```python
from build123d import *

# Parameters (mm, degrees)
SKETCH1_W                          = 165.1
SKETCH1_H                          = 12.7
BOSS_EXTRUDE1_DEPTH                = 127
SKETCH2_R                          = 30.63494
CUT_EXTRUDE1_DEPTH                 = 153.002606886
SKETCH3_R                          = 31.75
CUT_EXTRUDE2_DEPTH                 = 7.62
CUT_EXTRUDE3_DEPTH                 = 153.002606886
FILLET1_R                          = 3.175
FILLET2_R                          = 1.5875
SKETCH5_W                          = 101.6
SKETCH5_H                          = 9.525
CUT_EXTRUDE4_DEPTH                 = 153.002606886
FILLET3_R                          = 3.175
F_1_16_0_0625_DIAMETER_HOLE1_D     = 1.5875
F_1_16_0_0625_DIAMETER_HOLE1_DEPTH = 15.875
F_1_16_0_0625_DIAMETER_HOLE1_TIP   = 0.476933116
F_1_16_0_0625_DIAMETER_HOLE2_D     = 1.5875
F_1_16_0_0625_DIAMETER_HOLE2_DEPTH = 15.875
F_1_16_0_0625_DIAMETER_HOLE2_TIP   = 0.476933116
CUT_EXTRUDE5_DEPTH                 = 153.002606886


with BuildPart() as part:
    # Sketch1 → Boss-Extrude1 (new, symmetric)
    with BuildSketch(Plane(origin=(0, 0, 0), x_dir=(1, 0, 0), z_dir=(0, 1, 0))):
        Rectangle(SKETCH1_W, SKETCH1_H)
    extrude(amount=BOSS_EXTRUDE1_DEPTH, both=True)

    # Sketch2 → Cut-Extrude1 (cut, through all)
    with BuildSketch(Plane.XY.offset(6.35)):
        with Locations((0, 127)):
            Circle(SKETCH2_R)
    extrude(amount=-CUT_EXTRUDE1_DEPTH, mode=Mode.SUBTRACT)

    # Sketch3 → Cut-Extrude2 (cut)
    with BuildSketch(Plane(origin=(0, 0, -6.35), x_dir=(-1, 0, 0), z_dir=(0, 0, -1))):
        with Locations((0, 127)):
            Circle(SKETCH3_R)
    extrude(amount=-CUT_EXTRUDE2_DEPTH, mode=Mode.SUBTRACT)

    # Sketch4 → Cut-Extrude3 (cut, through all)
    with BuildSketch(Plane.XY.offset(6.35)):
        with BuildLine():
            Line((57.277, 127), (57.277, 104.775))
            Line((57.277, 104.775), (43.877983689, 104.775))
            Line((43.877983689, 104.775), (38.415383769, 114.236500603))
            ThreePointArc((38.415383769, 114.236500603), (39.624000301, 118.747116057), (44.134615883, 117.5385))
            Line((44.134615883, 117.5385), (47.690804866, 111.379))
            Line((47.690804866, 111.379), (50.673, 111.379))
            Line((50.673, 111.379), (50.673, 127))
            Line((50.673, 127), (57.277, 127))
        make_face()
        with BuildLine():
            Line((-50.673, 127), (-57.277, 127))
            Line((-57.277, 127), (-57.277, 104.775))
            Line((-57.277, 104.775), (-43.877983689, 104.775))
            Line((-43.877983689, 104.775), (-38.415383769, 114.236500603))
            ThreePointArc((-38.415383769, 114.236500603), (-39.624000301, 118.747116057), (-44.134615883, 117.5385))
            Line((-44.134615883, 117.5385), (-47.690804866, 111.379))
            Line((-47.690804866, 111.379), (-50.673, 111.379))
            Line((-50.673, 111.379), (-50.673, 127))
        make_face()
    extrude(amount=-CUT_EXTRUDE3_DEPTH, mode=Mode.SUBTRACT)

    # Fillet1
    fillet1_edges = [part.edges().sort_by_distance(p)[0] for p in [
        (50.673, 127, 0),
        (57.277, 127, 0),
        (57.277, 104.775, 0),
        (43.877983689, 104.775, 0),
        (-43.877983689, 104.775, 0),
        (-57.277, 104.775, 0),
        (-57.277, 127, 0),
        (-50.673, 127, 0),
    ]]
    fillet(fillet1_edges, radius=FILLET1_R)

    # Fillet2
    fillet2_edges = [part.edges().sort_by_distance(p)[0] for p in [
        (47.690804866, 111.379, 0),
        (50.673, 111.379, 0),
        (-50.673, 111.379, 0),
        (-47.690804866, 111.379, 0),
    ]]
    fillet(fillet2_edges, radius=FILLET2_R)

    # Sketch5 → Cut-Extrude4 (cut, through all)
    with BuildSketch(Plane.XY.offset(6.35)):
        with Locations((0, -122.2375)):
            Rectangle(SKETCH5_W, SKETCH5_H)
    extrude(amount=-CUT_EXTRUDE4_DEPTH, mode=Mode.SUBTRACT)

    # Fillet3
    fillet3_edges = [part.edges().sort_by_distance(p)[0] for p in [
        (-50.8, -127, 0),
        (-50.8, -117.475, 0),
        (50.8, -117.475, 0),
        (50.8, -127, 0),
    ]]
    fillet(fillet3_edges, radius=FILLET3_R)

    # 1/16 (0.0625) Diameter Hole1
    with Locations(Plane(origin=(82.55, 0, 0), x_dir=(0, 0, -1), z_dir=(1, 0, 0))):
        with Locations((0, -120.65), (0, -95.25), (0, 44.45), (0, 69.85), (0, 120.65)):
            Hole(F_1_16_0_0625_DIAMETER_HOLE1_D / 2, depth=F_1_16_0_0625_DIAMETER_HOLE1_DEPTH)
            with Locations((0, 0, -(F_1_16_0_0625_DIAMETER_HOLE1_DEPTH + F_1_16_0_0625_DIAMETER_HOLE1_TIP / 2))):  # 118° drill point
                Cone(0, F_1_16_0_0625_DIAMETER_HOLE1_D / 2, F_1_16_0_0625_DIAMETER_HOLE1_TIP, mode=Mode.SUBTRACT)

    # 1/16 (0.0625) Diameter Hole2
    with Locations(Plane.ZY.offset(82.55)):
        with Locations((0, -120.65), (0, -95.25), (0, 44.45), (0, 69.85), (0, 120.65)):
            Hole(F_1_16_0_0625_DIAMETER_HOLE2_D / 2, depth=F_1_16_0_0625_DIAMETER_HOLE2_DEPTH)
            with Locations((0, 0, -(F_1_16_0_0625_DIAMETER_HOLE2_DEPTH + F_1_16_0_0625_DIAMETER_HOLE2_TIP / 2))):  # 118° drill point
                Cone(0, F_1_16_0_0625_DIAMETER_HOLE2_D / 2, F_1_16_0_0625_DIAMETER_HOLE2_TIP, mode=Mode.SUBTRACT)

    # Sketch10 → Cut-Extrude5 (cut, through all)
    with BuildSketch(Plane.XY.offset(6.35)):
        with BuildLine():
            Line((-61.89437725, -88.484920775), (-50.783316982, 38.515079225))
            ThreePointArc((-50.783316982, 38.515079225), (-45.623860507, 42.84437725), (-41.294562483, 37.684920775))
            Line((-41.294562483, 37.684920775), (-52.40562275, -89.315079225))
            ThreePointArc((-52.40562275, -89.315079225), (-57.565079225, -93.64437725), (-61.89437725, -88.484920775))
        make_face()
        with BuildLine():
            Line((-27.00562275, -89.315079225), (-15.894562483, 37.684920775))
            ThreePointArc((-15.894562483, 37.684920775), (-20.223860507, 42.84437725), (-25.383316982, 38.515079225))
            Line((-25.383316982, 38.515079225), (-36.49437725, -88.484920775))
            ThreePointArc((-36.49437725, -88.484920775), (-32.165079225, -93.64437725), (-27.00562275, -89.315079225))
        make_face()
        with BuildLine():
            Line((-1.60562275, -89.315079225), (9.505437517, 37.684920775))
            ThreePointArc((9.505437517, 37.684920775), (5.176139493, 42.84437725), (0.016683018, 38.515079225))
            Line((0.016683018, 38.515079225), (-11.09437725, -88.484920775))
            ThreePointArc((-11.09437725, -88.484920775), (-6.765079225, -93.64437725), (-1.60562275, -89.315079225))
        make_face()
        with BuildLine():
            Line((23.79437725, -89.315079225), (34.905437517, 37.684920775))
            ThreePointArc((34.905437517, 37.684920775), (30.576139493, 42.84437725), (25.416683018, 38.515079225))
            Line((25.416683018, 38.515079225), (14.30562275, -88.484920775))
            ThreePointArc((14.30562275, -88.484920775), (18.634920775, -93.64437725), (23.79437725, -89.315079225))
        make_face()
        with BuildLine():
            Line((49.19437725, -89.315079225), (60.305437517, 37.684920775))
            ThreePointArc((60.305437517, 37.684920775), (55.976139493, 42.84437725), (50.816683018, 38.515079225))
            Line((50.816683018, 38.515079225), (39.70562275, -88.484920775))
            ThreePointArc((39.70562275, -88.484920775), (44.034920775, -93.64437725), (49.19437725, -89.315079225))
        make_face()
    extrude(amount=-CUT_EXTRUDE5_DEPTH, mode=Mode.SUBTRACT)


solid = part.part
```
Build history of the part. All positions in model axes, mm. A direction names the side the tool comes from. Give positions to 0.01 mm unless a question says otherwise; leave off trailing zeros. Loops run counter-clockwise (first coordinate to the right, second up) from the corner with the lowest first, then second, coordinate; pieces in that order, holes last.
Item 1: Drill centre lines: line 1 (Y direction, x = -74.75, z = 0); line 2 (Z direction, x = -77, y = 120.65); line 3 (X direction, y = 5, z = 1). Where is each one in solid material? Low to high.
Answers follow:
line 1: y = -127 to -121.44, -119.86 to -96.04, -94.46 to 43.66, 45.24 to 69.06, 70.64 to 119.86, 121.44 to 127
line 2: z = -6.35 to -0.79, 0.79 to 6.35
line 3: x = -82.55 to -53.72, -44.15 to -28.32, -18.75 to -2.92, 6.65 to 22.48, 32.05 to 47.88, 57.45 to 82.55
Item 2: Pull direction Y, two halves, no side cores. Call faces 1 (the face through (40.72, 110.244, 0.089)), 2 (the face through (39, 127, 0)), 3 (the face through (82.55, 2, 0)): released by +Y, released by -Y, zero draft, split by the parting line, or undercut.
Answers follow:
face 1: undercut
face 2: released by +Y
face 3: zero draft
Item 3: Slice it at A-A, the plane y = -3. List the corners of the cut face in (x, z), and give its area (3 significant figures).
Answers follow:
outline: (-82.55, -6.35) - (-54.42, -6.35) - (-54.42, 6.35) - (-82.55, 6.35) - close; (-44.85, -6.35) - (-29.02, -6.35) - (-29.02, 6.35) - (-44.85, 6.35) - close; (-19.45, -6.35) - (-3.62, -6.35) - (-3.62, 6.35) - (-19.45, 6.35) - close; (5.95, -6.35) - (21.78, -6.35) - (21.78, 6.35) - (5.95, 6.35) - close; (31.35, -6.35) - (47.18, -6.35) - (47.18, 6.35) - (31.35, 6.35) - close; (56.75, -6.35) - (82.55, -6.35) - (82.55, 6.35) - (56.75, 6.35) - close
area: 1,490 mm2
Item 4: Flat gauge pins, fed straight in: pin 1 (1.4 mm diameter, centred on y = 44.45, z = 0, fed in from -X); pin 2 (2 mm diameter, centred on y = 69.85, z = 0, fed in from -X); pin 3 (1.3 mm diameter, centred on y = -95.25, z = 0, fed in from +X); pin 4 (3 mm diameter, centred on x = -30, z = 2, fed in from -Y) (3 decimals). Where does each tip first touch, or does it go through?
Answers follow:
pin 1: stops at x = -66.62
pin 2: stops at x = -82.55
pin 3: stops at x = 66.59
pin 4: stops at y = -117.475
Item 5: Which spindle directions (+Z, -Z, +X, -X, +Y, -Y) get a long thin tool onto all of the face, cutting with end or side? Do faces 4 (the face through (-82.55, 2, 0)), 5 (the face through (45.662, 114.893, 0.089)), 6 (the face through (-50.673, 118, 0)). Say none if no direction does.
Answers follow:
face 4: +Z, -Z, -X, +Y, -Y
face 5: +Z, -Z
face 6: +Z, -Z, +Y
